```python
from build123d import *

# Parameters (mm, degrees)
BOSS_EXTRUDE3_DEPTH      = 3.5
BOSS_EXTRUDE3_DEPTH_BACK = 3.5
SKETCH4_R                = 1.25
CUT_EXTRUDE1_DEPTH       = 3.5
SKETCH5_R                = 2.25
SKETCH5_R_2              = 1.25
BOSS_EXTRUDE5_DEPTH      = 0.5
SKETCH8_R                = 1.5
CUT_EXTRUDE3_DEPTH       = 47
SKETCH10_R               = 1.5
CUT_EXTRUDE4_DEPTH       = 47


with BuildPart() as part:
    # Sketch1 → Boss-Extrude3 (new body, two sides)
    with BuildSketch(Plane.XY) as boss_extrude3_sk:
        Polygon((-47, 0), (47, 0), (47, -12), (46.584070796, -12), (45.5, -12), (45.5, -1.5), (-45.5, -1.5), (-45.5, -12), (-47, -12), align=None)
    extrude(amount=BOSS_EXTRUDE3_DEPTH)
    extrude(boss_extrude3_sk.sketch, amount=-BOSS_EXTRUDE3_DEPTH_BACK)

    # Sketch4 → Cut-Extrude1 (cut)
    with BuildSketch(Plane(origin=(0, 0, 0), x_dir=(1, 0, 0), z_dir=(0, 1, 0))):
        Circle(SKETCH4_R)
    extrude(amount=-CUT_EXTRUDE1_DEPTH, mode=Mode.SUBTRACT)

    # Sketch5 → Boss-Extrude5 (add)
    with BuildSketch(Plane(origin=(0, 0, 0), x_dir=(1, 0, 0), z_dir=(0, 1, 0))):
        Circle(SKETCH5_R)
        Circle(SKETCH5_R_2, mode=Mode.SUBTRACT)
    extrude(amount=BOSS_EXTRUDE5_DEPTH)

    # Sketch8 → Cut-Extrude3 (cut)
    with BuildSketch(Plane(origin=(0, 0, 0), x_dir=(0, 0, -1), z_dir=(1, 0, 0))):
        with Locations((0, -8)):
            Circle(SKETCH8_R)
    extrude(amount=CUT_EXTRUDE3_DEPTH, mode=Mode.SUBTRACT)

    # Sketch10 → Cut-Extrude4 (cut)
    with BuildSketch(Plane(origin=(0, 0, 0), x_dir=(0, 0, -1), z_dir=(1, 0, 0))):
        with Locations((0, -8)):
            Circle(SKETCH10_R)
    extrude(amount=-CUT_EXTRUDE4_DEPTH, mode=Mode.SUBTRACT)


solid = part.part
```
Verification items for the finished model (mm, model axes). A direction names the side the tool comes from. Round coordinates to 2 decimals unless told otherwise and drop trailing zeros. Order: outer loops, then holes, each group sorted by start corner. A loop starts at its lowest first (then second) coordinate and runs counter-clockwise, first axis right, second up. Notation, with made-up numbers: (-4, -24) - (14, -24) arc R22 ccw to (14, 4) - close; hole circle Ø6 at (-35, 62). An arc over 180 degrees is marked (long way). Use CSV: the item, a comma, the result in double quotes. Start each with the question number.
1) Go/stop test with flat-tipped pins: P1, Ø4, axis at x = -20.5, z = -0.5, coming from the +Y side; P2, Ø1, axis at x = -35, z = 1.5, coming from the -Y side; P3, Ø1.5, axis at x = 0, z = 0, coming from the -Y side. Record where each tip stops, or that it passes through.
2) Thickness scan on L1, parallel to X at y = -4, z = 3; L2, parallel to Z at x = 0, y = 0.2; L3, parallel to X at y = -0.9, z = 0. Record the ranges inside material, lowest first.
3) Section check C-C, the plane y = -3. Record the cut outline in (x, z).
4) Access from +Z, -Z, +X, -X, +Y, -Y to the whole of each face (thin tool, end or side, straight path). Record for faces 1 (the flat face through (46, -12, 0)), 2 (the flat face through (-45.5, -6, 0)), 3 (the cylindrical face through (-0.29, 0.25, -2.23)).
5) Mould release check, pull along Z, two halves, no side actions. Record for faces 4 (the flat face through (-46, -12, 0)), 5 (the cylindrical face through (-46.24, -9.464, 0.325)), 6 (the flat face through (0, -1, -3.5)): +Z half, -Z half, draft (parallel to the pull), parting line (faces both ways), or undercut.
6) Section check A-A, the plane y = -8. Record the cut outline in (x, z), plus the area to 3 significant figures.
7) Section check D-D, the plane x = 0. Record the cut outline in (y, z).
8) Section check B-B, the plane z = 0. Record the cut outline in (x, y).
Answers:
1,P1,"stops at y = 0"
1,P2,"stops at y = -1.5"
1,P3,"passes through"
2,L1,"x = -47 to -45.5, 45.5 to 47"
2,L2,"z = -2.25 to -1.25, 1.25 to 2.25"
2,L3,"x = -47 to -1.25, 1.25 to 47"
3,outline,"(-47, -3.5) - (-45.5, -3.5) - (-45.5, 3.5) - (-47, 3.5) - close; (45.5, -3.5) - (47, -3.5) - (47, 3.5) - (45.5, 3.5) - close"
4,face 1,"+Z, -Z, +X, -X, -Y"
4,face 2,"+Z, -Z, -Y"
4,face 3,"+Y"
5,face 4,"draft"
5,face 5,"undercut"
5,face 6,"-Z half"
6,outline,"(-47, -3.5) - (-45.5, -3.5) - (-45.5, -1.5) - (-47, -1.5) - close; (-47, 1.5) - (-45.5, 1.5) - (-45.5, 3.5) - (-47, 3.5) - close; (45.5, -3.5) - (47, -3.5) - (47, -1.5) - (45.5, -1.5) - close; (45.5, 1.5) - (47, 1.5) - (47, 3.5) - (45.5, 3.5) - close"
6,area,"12.0 mm²"
7,outline,"(-1.5, -3.5) - (0, -3.5) - (0, -2.25) - (0.5, -2.25) - (0.5, -1.25) - (-1.5, -1.25) - close; (-1.5, 1.25) - (0.5, 1.25) - (0.5, 2.25) - (0, 2.25) - (0, 3.5) - (-1.5, 3.5) - close"
8,outline,"(-47, -12) - (-45.5, -12) - (-45.5, -9.5) - (-47, -9.5) - close; (-47, -6.5) - (-45.5, -6.5) - (-45.5, -1.5) - (-1.25, -1.5) - (-1.25, 0.5) - (-2.25, 0.5) - (-2.25, 0) - (-47, 0) - close; (1.25, -1.5) - (45.5, -1.5) - (45.5, -6.5) - (47, -6.5) - (47, 0) - (2.25, 0) - (2.25, 0.5) - (1.25, 0.5) - close; (45.5, -12) - (47, -12) - (47, -9.5) - (45.5, -9.5) - close"
